Here's how the part is built. I have some questions about the finished solid (model axes, mm). A direction names the side the tool comes from. Give positions to 0.01 mm unless a question says otherwise; leave off trailing zeros. Loops run counter-clockwise (first coordinate to the right, second up) from the corner with the lowest first, then second, coordinate; pieces in that order, holes last.
Q1. If we section it at D-D (y = 1): Please give me the cut outline in (x, z).
Q2. Will these pins go through, and if not, where does the flat tip stop? P1, Ø1.5, axis at x = 7, z = -2, coming from the -Y side; P2, Ø3, axis at x = -1, y = -5.5, coming from the -Z side; P3, Ø0.8, axis at y = -1, z = -12, coming from the -X side.
Q3. I need wall thicknesses on line 1 (X direction, y = 0.7, z = -11); line 2 (Z direction, x = 10.25, y = 0.5); line 3 (Y direction, x = -2.25, z = 6.75). Which ranges of each line are inside material? Lowest first, please.
Q4. We'd pull the mould along Z, two halves only. Please class faces 5 (the face through (-11.5, 0.76, 10.55)), 6 (the face through (-12.25, 2, 0)), 7 (the face through (0.028, 2.199, 12.965)), 8 (the face through (11, 1, -12)): +Z half, -Z half, draft (parallel to the pull), parting line (faces both ways), or undercut.
Q5. If we section it at A-A (x = 10.25): Please give me the cut outline in (y, z), plus the area to 4 significant figures.
Q6. For faces 1 (the face through (2, 2, 11)), 2 (the face through (0, 1.5, -9)), 3 (the face through (-5, -1, -12)), 4 (the face through (12.25, 2, 0)), which set-ups out of +Z, -Z, +X, -X, +Y, -Y let a thin tool reach every point of the face, with its end or its side?
Q7. If we section it at B-B (z = 10.6): Please give me the cut outline in (x, y), plus the area to 3 significant figures.
Q8. If we section it at C-C (y = -1.5): Please give me the cut outline in (x, z).
from build123d import *

# Parameters (mm, degrees)
SKETCH1_W                  = 25
SKETCH1_H                  = 26.5
BOSS_EXTRUDE1_DEPTH        = 1.5
SKETCH2_W                  = 24.5
SKETCH2_H                  = 17
BOSS_EXTRUDE2_DEPTH        = 1.5
SKETCH3_R                  = 1.25
CUT_EXTRUDE1_DEPTH         = 7.5
SKETCH4_R                  = 1.25
CUT_EXTRUDE2_DEPTH         = 7.5
SKETCH5_W                  = 4
SKETCH5_H                  = 5
BOSS_EXTRUDE3_DEPTH        = 1
FILLET1_R                  = 1
BOSS_EXTRUDE4_START        = -9.6
SKETCH6_R                  = 0.25
BOSS_EXTRUDE4_DEPTH        = 10.6
CHAMFER1_SIZE              = 0.1
FILLET2_R                  = 0.5
LPATTERN1_COUNT            = 4
LPATTERN1_PITCH            = 2.54
CHAMFER1_OF_LPATTERN1_SIZE = 0.1
FILLET2_OF_LPATTERN1_R     = 0.5
SKETCH7_W                  = 10
SKETCH7_H                  = 2.5
BOSS_EXTRUDE5_DEPTH        = 2.5
FILLET3_R                  = 0.75


with BuildPart() as part:
    # Sketch1 → Boss-Extrude1 (new body)
    with BuildSketch(Plane(origin=(0, 0, 0), x_dir=(1, 0, 0), z_dir=(0, 1, 0))):
        Rectangle(SKETCH1_W, SKETCH1_H)
    extrude(amount=BOSS_EXTRUDE1_DEPTH)

    # Sketch2 → Boss-Extrude2 (add)
    with BuildSketch(Plane(origin=(0, 1.5, 0), x_dir=(1, 0, 0), z_dir=(0, 1, 0))):
        with Locations((0, 0.25)):
            Rectangle(SKETCH2_W, SKETCH2_H)
    extrude(amount=BOSS_EXTRUDE2_DEPTH)

    # Sketch3 → Cut-Extrude1 (cut)
    with BuildSketch(Plane(origin=(0, 1.5, 0), x_dir=(1, 0, 0), z_dir=(0, 1, 0))):
        with Locations((-10.25, -10.6)):
            Circle(SKETCH3_R)
    cut_extrude1 = extrude(amount=-CUT_EXTRUDE1_DEPTH, mode=Mode.SUBTRACT)

    # Mirror1: Cut-Extrude1 across plane
    add(cut_extrude1.mirror(Plane(origin=(0, 0, 0), x_dir=(0, 0, 1), z_dir=(1, 0, 0))), mode=Mode.SUBTRACT)

    # Sketch4 → Cut-Extrude2 (cut)
    with BuildSketch(Plane(origin=(0, 1.5, 0), x_dir=(1, 0, 0), z_dir=(0, 1, 0))):
        with Locations((-10.25, 11)):
            Circle(SKETCH4_R)
    cut_extrude2 = extrude(amount=-CUT_EXTRUDE2_DEPTH, mode=Mode.SUBTRACT)

    # Mirror2: Cut-Extrude2 across plane
    add(cut_extrude2.mirror(Plane(origin=(0, 0, 0), x_dir=(0, 0, 1), z_dir=(1, 0, 0))), mode=Mode.SUBTRACT)

    # Sketch5 → Boss-Extrude3 (add)
    with BuildSketch(Plane(origin=(0, 1.5, 0), x_dir=(1, 0, 0), z_dir=(0, 1, 0))):
        with Locations((0, -10.75)):
            Rectangle(SKETCH5_W, SKETCH5_H)
    extrude(amount=BOSS_EXTRUDE3_DEPTH)

    # Fillet1
    fillet1_edges = [part.edges().sort_by_distance(p)[0] for p in [
        (0, 2.5, 13.25),
    ]]
    fillet(fillet1_edges, radius=FILLET1_R)

    # Sketch6 → Boss-Extrude4 (add)
    with BuildSketch(Plane(origin=(0, 1.5, 0), x_dir=(1, 0, 0), z_dir=(0, 1, 0)).offset(BOSS_EXTRUDE4_START)):
        with Locations((-3.81, 12)):
            Circle(SKETCH6_R)
    boss_extrude4 = extrude(amount=BOSS_EXTRUDE4_DEPTH)

    # Chamfer1
    chamfer1_edges = [part.edges().sort_by_distance(p)[0] for p in [
        (-4.06, 2.5, -12),
    ]]
    chamfer(chamfer1_edges, length=CHAMFER1_SIZE)

    # Fillet2
    fillet2_edges = [part.edges().sort_by_distance(p)[0] for p in [
        (-4.06, 1.5, -12),
    ]]
    fillet(fillet2_edges, radius=FILLET2_R)

    # LPattern1: Boss-Extrude4 ×4
    with Locations(*[(i * LPATTERN1_PITCH, 0, 0) for i in range(1, LPATTERN1_COUNT)]):
        add(boss_extrude4)

    # Chamfer1 of LPattern1
    chamfer1_of_lpattern1_edges = [part.edges().sort_by_distance(p)[0] for p in [
        (-1.52, 2.5, -12),
        (1.02, 2.5, -12),
        (3.56, 2.5, -12),
    ]]
    chamfer(chamfer1_of_lpattern1_edges, length=CHAMFER1_OF_LPATTERN1_SIZE)

    # Fillet2 of LPattern1
    fillet2_of_lpattern1_edges = [part.edges().sort_by_distance(p)[0] for p in [
        (-1.52, 1.5, -12),
        (1.02, 1.5, -12),
        (3.56, 1.5, -12),
    ]]
    fillet(fillet2_of_lpattern1_edges, radius=FILLET2_OF_LPATTERN1_R)

    # Sketch7 → Boss-Extrude5 (add)
    with BuildSketch(Plane.XZ):
        with Locations((0, -12)):
            Rectangle(SKETCH7_W, SKETCH7_H)
    extrude(amount=BOSS_EXTRUDE5_DEPTH)

    # Fillet3
    fillet3_edges = [part.edges().sort_by_distance(p)[0] for p in [
        (-5, -1.25, -10.75),
        (-5, -1.25, -13.25),
        (5, -1.25, -13.25),
        (5, -1.25, -10.75),
    ]]
    fillet(fillet3_edges, radius=FILLET3_R)


solid = part.part
Check sheet entries:
1. outline: (-12.5, -13.25) - (12.5, -13.25) - (12.5, 13.25) - (-12.5, 13.25) - close; hole circle Ø2.5 at (-10.25, -11); hole circle Ø2.5 at (-10.25, 10.6); hole circle Ø2.5 at (10.25, -11); hole circle Ø2.5 at (10.25, 10.6)
2. P1: stops at y = 0
2. P2: stops at z = -12.25
2. P3: stops at x = -5
3. line 1: x = -12.5 to -11.5, -9 to 9, 11.5 to 12.5
3. line 2: z = -13.25 to -12.25, -9.75 to 9.35, 11.85 to 13.25
3. line 3: y = 0 to 3
4. face 5: undercut
4. face 6: draft
4. face 7: +Z half
4. face 8: undercut
5. outline: (0, -13.25) - (1.5, -13.25) - (1.5, -12.25) - (0, -12.25) - close; (0, -9.75) - (1.5, -9.75) - (1.5, -8.75) - (3, -8.75) - (3, 8.25) - (1.5, 8.25) - (1.5, 9.35) - (0, 9.35) - close; (0, 11.85) - (1.5, 11.85) - (1.5, 13.25) - (0, 13.25) - close
5. area: 57.75 mm2
6. face 1: +Z, +X, +Y
6. face 2: +Y
6. face 3: +Z, -Z, -X, -Y
6. face 4: +Z, -Z, +X, +Y
7. outline: (-12.5, 0) - (-11.5, 0) - (-11.5, 1.5) - (-12.5, 1.5) - close; (-9, 0) - (9, 0) - (9, 1.5) - (2, 1.5) - (2, 2.5) - (-2, 2.5) - (-2, 1.5) - (-9, 1.5) - close; (11.5, 0) - (12.5, 0) - (12.5, 1.5) - (11.5, 1.5) - close
7. area: 34.0 mm2
8. outline: (-5, -12.5) arc R0.75 ccw to (-4.25, -13.25) - (4.25, -13.25) arc R0.75 ccw to (5, -12.5) - (5, -11.5) arc R0.75 ccw to (4.25, -10.75) - (-4.25, -10.75) arc R0.75 ccw to (-5, -11.5) - close
